Here's how the part is built. I have some questions about the finished solid (model axes, mm). Face numbers are marked on the shaded views. A direction names the side the tool comes from. Round coordinates to 2 decimals unless told otherwise and drop trailing zeros. Order: outer loops, then holes, each group sorted by start corner. A loop starts at its lowest first (then second) coordinate and runs counter-clockwise, first axis right, second up. Notation, with made-up numbers: M 16.5,5 L 67.5,5 A25 ccw 67.5,39 Z; hole C 15.5,47 d9. An arc over 180 degrees is marked long. Write item = value, one per line. Start each with the question number.
Item 1: We'd pull the mould along X, two halves only. Please class the marked faces 3, 4 and 5: pulls with the +X half, pulls with the -X half, needs draft (parallel to the pull), parting line crosses it, or undercut.
Item 2: I'm going to push flat-ended pins straight in: P1, Ø1, axis at y = -1.5, z = 6.5, coming from the -X side; P2, Ø1.5, axis at x = 0.5, y = 0.5, coming from the -Z side; P3, Ø1, axis at x = 1.5, y = 1, coming from the -Z side; P4, Ø1, axis at y = 2, z = 4, coming from the +X side. Where does each tip first touch, or does it pass through?
Item 3: For the marked faces 1 and 2, which set-ups out of +Z, -Z, +X, -X, +Y, -Y let a thin tool reach every point of the face, with its end or its side?
Item 4: I want a section at D-D, the plane y = -0.9. List the corners of the cut face in (x, z) for me, plus the area to 3 significant figures.
Item 5: I want a section at A-A, the plane z = 1.25. List the corners of the cut face in (x, y) for me, plus the area to 3 significant figures.
Item 6: I want a section at C-C, the plane z = 8.75. List the corners of the cut face in (x, y) for me, plus the area to 3 significant figures.
Item 7: Please list where these lines run through material, in increasing order: L1, parallel to Y at x = 0, z = 1.8; L2, parallel to Z at x = 0.35, y = -1.95; L3, parallel to Z at x = -0.2, y = 0.3.
Item 8: I want a section at B-B, the plane x = 0. List the corners of the cut face in (y, z) for me, plus the area to 3 significant figures.
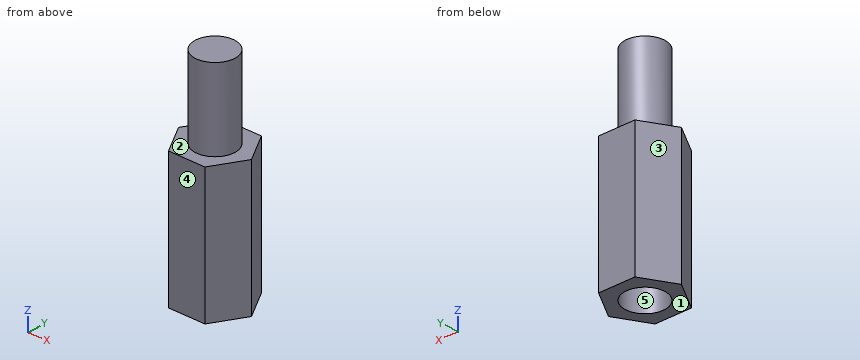
```python
from build123d import *

# Parameters (mm, degrees)
EXTRUDE_1_DEPTH     = 10
SKETCH_2_R          = 1.5
EXTRUDE_2_DEPTH     = 6
SKETCH_3_R          = 1.5
CUT_EXTRUDE_1_DEPTH = 6


with BuildPart() as part:
    # 草图1 → 凸台-拉伸1 (new body)
    with BuildSketch(Plane.XY):
        Polygon((2.713546265, 0), (1.356773133, 2.35), (-1.356773133, 2.35), (-2.713546265, 0), (-1.356773133, -2.35), (1.356773133, -2.35), align=None)
    extrude(amount=EXTRUDE_1_DEPTH)

    # 草图2 → 凸台-拉伸2 (add)
    with BuildSketch(Plane.XY.offset(10)):
        Circle(SKETCH_2_R)
    extrude(amount=EXTRUDE_2_DEPTH)

    # 草图3 → 切除-拉伸1 (cut)
    with BuildSketch(Plane(origin=(0, 0, 0), x_dir=(-1, 0, 0), z_dir=(0, 0, -1))):
        with Locations(Location((0, 0, 0), (0, 0, 180))):
            Circle(SKETCH_3_R)
    extrude(amount=-CUT_EXTRUDE_1_DEPTH, mode=Mode.SUBTRACT)


solid = part.part
```
Filled in:
q1.face_3 = pulls with the -X half
q1.face_4 = needs draft
q1.face_5 = undercut
q2.P1 = -2.14
q2.P2 = 6
q2.P3 = 0
q2.P4 = 1.85
q3.face_1 = -Z, +X, -X, +Y, -Y
q3.face_2 = +Z
q4.outline = M -2.19,0 L -1.2,0 L -1.2,6 L 1.2,6 L 1.2,0 L 2.19,0 L 2.19,10 L 1.2,10 L 1.2,16 L -1.2,16 L -1.2,10 L -2.19,10 Z
q4.area = 43.9 mm^2
q5.outline = M -2.71,0 L -1.36,-2.35 L 1.36,-2.35 L 2.71,0 L 1.36,2.35 L -1.36,2.35 Z; hole C 0,0 d3
q5.area = 12.1 mm^2
q6.outline = M -2.71,0 L -1.36,-2.35 L 1.36,-2.35 L 2.71,0 L 1.36,2.35 L -1.36,2.35 Z
q6.area = 19.1 mm^2
q7.L1 = -2.35 to -1.5, 1.5 to 2.35
q7.L2 = 0 to 10
q7.L3 = 6 to 16
q8.outline = M -2.35,0 L -1.5,0 L -1.5,6 L 1.5,6 L 1.5,0 L 2.35,0 L 2.35,10 L 1.5,10 L 1.5,16 L -1.5,16 L -1.5,10 L -2.35,10 Z
q8.area = 47.0 mm^2
